Check sheet for the modelled part. Datum: model origin and axes. Units: mm. A direction names the side the tool comes from. Round coordinates to 2 decimals unless told otherwise and drop trailing zeros. Order: outer loops, then holes, each group sorted by start corner. A loop starts at its lowest first (then second) coordinate and runs counter-clockwise, first axis right, second up.
Q1. Cross-section at C-C on z = 55.5. Record the cut outline in (x, y).
Q2. Cross-section at B-B on y = 4.25. Give the number of separate pieces and of enclosed holes in the cut face, then the cut area to 3 significant figures.
Q3. Cross-section at A-A on x = 50. Record the cut outline in (y, z).
Q4. Depth check by flat-ended pin: P1, Ø5, axis at x = 102, z = -65, coming from the -Y side; P2, Ø2.5, axis at y = 3.5, z = -64.5, coming from the -X side; P3, Ø2, axis at x = 145, y = 2.5, coming from the -Z side. Enter the tip coordinate at first touch or a pass-through.
Q5. Set-up check for faces 4 (the flat face through (34, 5, -47.25)), 5 (the flat face through (15, 4, 90)), 6 (the flat face through (26, 4, -61.5)): record each of +Z, -Z, +X, -X, +Y, -Y from which the full face is reachable in a straight line by a thin tool's end or side.
Q6. Scan lines: probe 1 along Z at (x, y) = (68, 7.75); probe 2 along Z at (x, y) = (-16, 2.25); probe 3 along X at (y, z) = (6.5, -80). Record each from-to range of solid material in increasing order.
Q7. Mould release check, pull along X, two halves, no side actions. Record for faces 1 (the flat face through (-87, 4, 62)), 2 (the flat face through (43, 0, 61)), 3 (the flat face through (66.45, 4, 67)): +X half, -X half, draft (parallel to the pull), parting line (faces both ways), or undercut.
from build123d import *

# Parameters (mm, degrees)
SALIENTE_EXTRUIR1_DEPTH = 8
CROQUIS2_R              = 1.825
CROQUIS2_W              = 80.45
CROQUIS2_H              = 10
CORTAR_EXTRUIR1_DEPTH   = 220.463870727
CROQUIS3_R              = 1.825
CORTAR_EXTRUIR2_DEPTH   = 220.463870727
CROQUIS4_W              = 106.5
CROQUIS4_H              = 94.5
CORTAR_EXTRUIR3_DEPTH   = 6.5
REDONDEO1_R             = 2.3
CROQUIS5_R              = 1.825
CORTAR_EXTRUIR4_DEPTH   = 220.463870727
CROQUIS6_W              = 102.5
CROQUIS6_H              = 90.5
CORTAR_EXTRUIR5_DEPTH   = 220.414312556
CROQUIS9_R              = 1.825
CORTAR_EXTRUIR7_DEPTH   = 220.463870727
CROQUIS11_R             = 1.825
CORTAR_EXTRUIR8_DEPTH   = 220.463870727


with BuildPart() as part:
    # Croquis1 → Saliente-Extruir1 (new body)
    with BuildSketch(Plane(origin=(0, 0, 0), x_dir=(1, 0, 0), z_dir=(0, 1, 0))):
        with BuildLine():
            Line((0, 0), (200, 0))
            Line((200, 0), (200, 15.2))
            ThreePointArc((200, 15.2), (197.701163079, 20.938172036), (191.9990235, 23.3249845))
            ThreePointArc((191.9990235, 23.3249845), (148.666739026, 44.032184001), (120.7781513, 83.1307986))
            ThreePointArc((120.7781513, 83.1307986), (113.982057966, 88.196272982), (105.7, 90))
            Line((105.7, 90), (0, 90))
            Line((0, 90), (-79, 90))
            ThreePointArc((-79, 90), (-84.638146896, 87.675499941), (-86.999825594, 82.052824894))
            Line((-86.999825594, 82.052824894), (-86.999825594, 41.494023494))
            ThreePointArc((-86.999825594, 41.494023494), (-92.052704294, 29.329564667), (-102.353503833, 21.119864881))
            ThreePointArc((-102.353503833, 21.119864881), (-108.040391417, 18.79326931), (-110.4, 13.12))
            Line((-110.4, 13.12), (-110.4, 0))
            Line((-110.4, 0), (0, 0))
        make_face()
    extrude(amount=SALIENTE_EXTRUIR1_DEPTH)

    # Simetría2: part across plane


with BuildPart() as part_1:
    add(part.part)
    add(part.part.mirror(Plane(origin=(0, 8, 0), x_dir=(1, 0, 0), z_dir=(0, 0, -1))))

    # Croquis2 → Cortar-Extruir1 (cut, through all)
    with BuildSketch(Plane(origin=(0, 8, 0), x_dir=(1, 0, 0), z_dir=(0, 1, 0))):
        with Locations(Location((68.5, 81.35, 0), (0, 0, 270))):
            Circle(CROQUIS2_R)
        with Locations(Location((-16.05, 81.35, 0), (0, 0, 270))):
            Circle(CROQUIS2_R)
        with Locations(Location((68.5, -81.35, 0), (0, 0, 90))):
            Circle(CROQUIS2_R)
        with Locations(Location((-16.05, -81.35, 0), (0, 0, 90))):
            Circle(CROQUIS2_R)
        with Locations((26.225, -66.5)):
            Rectangle(CROQUIS2_W, CROQUIS2_H)
        with Locations((26.225, 66.5)):
            Rectangle(CROQUIS2_W, CROQUIS2_H)
    extrude(amount=-CORTAR_EXTRUIR1_DEPTH, mode=Mode.SUBTRACT)

    # Croquis3 → Cortar-Extruir2 (cut, through all)
    with BuildSketch(Plane(origin=(0, 8, 0), x_dir=(1, 0, 0), z_dir=(0, 1, 0))):
        with Locations(Location((-76.999825594, -46.75, 0), (0, 0, 270))):
            Circle(CROQUIS3_R)
        with Locations(Location((-34.999825594, -46.75, 0), (0, 0, 270))):
            Circle(CROQUIS3_R)
        with Locations(Location((-34.999825594, 46.75, 0), (0, 0, 90))):
            Circle(CROQUIS3_R)
        with Locations(Location((-76.999825594, 46.75, 0), (0, 0, 90))):
            Circle(CROQUIS3_R)
    extrude(amount=-CORTAR_EXTRUIR2_DEPTH, mode=Mode.SUBTRACT)

    # Croquis4 → Cortar-Extruir3 (cut)
    with BuildSketch(Plane(origin=(0, 8, 0), x_dir=(1, 0, 0), z_dir=(0, 1, 0))):
        with Locations((34.525174406, 0)):
            Rectangle(CROQUIS4_W, CROQUIS4_H)
    extrude(amount=-CORTAR_EXTRUIR3_DEPTH, mode=Mode.SUBTRACT)

    # Redondeo1
    redondeo1_edges = [part_1.edges().sort_by_distance(p)[0] for p in [
        (87.775174406, 4.75, -47.25),
        (87.775174406, 4.75, 47.25),
        (-18.724825594, 4.75, 47.25),
        (-18.724825594, 4.75, -47.25),
    ]]
    fillet(redondeo1_edges, radius=REDONDEO1_R)

    # Croquis5 → Cortar-Extruir4 (cut, through all)
    with BuildSketch(Plane(origin=(0, 8, 0), x_dir=(1, 0, 0), z_dir=(0, 1, 0))):
        with Locations(Location((98.35, 28.84, 0), (0, 0, 270))):
            Circle(CROQUIS5_R)
        with Locations(Location((98.35, -28.84, 0), (0, 0, 90))):
            Circle(CROQUIS5_R)
        with Locations(Location((164.35, 11.66, 0), (0, 0, 270))):
            Circle(CROQUIS5_R)
        with Locations(Location((164.35, -11.66, 0), (0, 0, 90))):
            Circle(CROQUIS5_R)
    extrude(amount=-CORTAR_EXTRUIR4_DEPTH, mode=Mode.SUBTRACT)

    # Croquis6 → Cortar-Extruir5 (cut, through all)
    with BuildSketch(Plane(origin=(0, 1.5, 0), x_dir=(1, 0, 0), z_dir=(0, 1, 0))):
        with Locations((34.525174406, 0)):
            Rectangle(CROQUIS6_W, CROQUIS6_H)
    extrude(amount=-CORTAR_EXTRUIR5_DEPTH, mode=Mode.SUBTRACT)

    # Croquis9 → Cortar-Extruir7 (cut, through all)
    with BuildSketch(Plane(origin=(0, 8, 0), x_dir=(1, 0, 0), z_dir=(0, 1, 0))):
        with Locations(Location((-80.675393895, -75.767215538, 0), (0, 0, 270))):
            Circle(CROQUIS9_R)
        with Locations(Location((-58.52366486, -80.370640978, 0), (0, 0, 270))):
            Circle(CROQUIS9_R)
        with Locations(Location((-58.52366486, 80.370640978, 0), (0, 0, 90))):
            Circle(CROQUIS9_R)
        with Locations(Location((-80.675393895, 75.767215538, 0), (0, 0, 90))):
            Circle(CROQUIS9_R)
    extrude(amount=-CORTAR_EXTRUIR7_DEPTH, mode=Mode.SUBTRACT)

    # Croquis11 → Cortar-Extruir8 (cut, through all)
    with BuildSketch(Plane(origin=(0, 8, 0), x_dir=(1, 0, 0), z_dir=(0, 1, 0))):
        with Locations(Location((-58.4, 46.75, 0), (0, 0, 270))):
            Circle(CROQUIS11_R)
        with Locations(Location((-58.4, -46.75, 0), (0, 0, 90))):
            Circle(CROQUIS11_R)
    extrude(amount=-CORTAR_EXTRUIR8_DEPTH, mode=Mode.SUBTRACT)


solid = part_1.part
Results found:
1. outline: (-87, 0) - (137.15, 0) - (137.15, 8) - (-87, 8) - close
2. separate pieces: 1
2. enclosed holes: 21
2. area: 33,000 mm2
3. outline: (0, -90) - (8, -90) - (8, -71.5) - (0, -71.5) - close; (0, -61.5) - (8, -61.5) - (8, -47.25) - (1.5, -47.25) - (1.5, -45.25) - (0, -45.25) - close; (0, 45.25) - (1.5, 45.25) - (1.5, 47.25) - (8, 47.25) - (8, 61.5) - (0, 61.5) - close; (0, 71.5) - (8, 71.5) - (8, 90) - (0, 90) - close
4. P1: stops at y = 0
4. P2: stops at x = -87
4. P3: stops at z = -48.22
5. face 4: +Y
5. face 5: +Z, +X, -X, +Y, -Y
5. face 6: +Y, -Y
6. probe 1: z = -90 to -83.11, -79.59 to -47.25, 47.25 to 79.59, 83.11 to 90
6. probe 2: z = -90 to -83.17, -79.53 to -47.25, 47.25 to 79.53, 83.17 to 90
6. probe 3: x = -87 to -60.31, -56.74 to -17.28, -14.82 to 67.27, 69.73 to 122.04
7. face 1: -X half
7. face 2: draft
7. face 3: undercut
